Here's how the part is built. I have some questions about the finished solid (model axes, mm). A direction names the side the tool comes from. Give positions to 0.01 mm unless a question says otherwise; leave off trailing zeros. Write each loop counter-clockwise with the first axis right and the second up, starting at its lowest first coordinate (ties: lowest second). Pieces come first, ordered by that corner, then holes. Notation, with made-up numbers: (41, 24.25) - (83, 24.25) arc R24 ccw to (83, 39.25) - close; hole circle Ø11 at (56.25, 40.5). An arc over 180 degrees is marked (long way). Use a Markdown table: item, result.
```python
from build123d import *

# Parameters (mm, degrees)
SKETCH1_R               = 14.95
BOSS_EXTRUDE1_DEPTH     = 14
SKETCH3_R               = 14.95
BOSS_EXTRUDE2_DEPTH     = 14
CHAMFER1_SIZE           = 1
SKETCH11_R              = 11.5
BOSS_EXTRUDE3_DEPTH     = 9
CUT_EXTRUDE1_DEPTH      = 37.465120321
CUT_EXTRUDE1_DEPTH_BACK = 37.465120321
SKETCH9_R               = 7.2
CUT_EXTRUDE2_DEPTH      = 37.465120321
CUT_EXTRUDE2_DEPTH_BACK = 37.465120321
SKETCH10_W              = 2.718236021
SKETCH10_H              = 5.3


with BuildPart() as part:
    # Sketch1 → Boss-Extrude1 (new body)
    with BuildSketch(Plane(origin=(0, 0, 0), x_dir=(1, 0, 0), z_dir=(0, 1, 0))):
        with Locations(Location((0, 0, 0), (0, 0, 270))):
            Circle(SKETCH1_R)
    extrude(amount=BOSS_EXTRUDE1_DEPTH)

    # Sketch3 → Boss-Extrude2 (add)
    with BuildSketch(Plane.XZ):
        with Locations(Location((3, 0, 0), (0, 0, 95.758429808))):
            Circle(SKETCH3_R)
    extrude(amount=BOSS_EXTRUDE2_DEPTH)

    # Chamfer1
    chamfer1_edges = [part.edges().sort_by_distance(p)[0] for p in [
        (0, 14, -14.95),
        (4.5, -14, -14.874558817),
    ]]
    chamfer(chamfer1_edges, length=CHAMFER1_SIZE)

    # Sketch11 → Boss-Extrude3 (add)
    with BuildSketch(Plane(origin=(0, 14, 0), x_dir=(1, 0, 0), z_dir=(0, 1, 0))):
        with Locations(Location((1.5, 0, 0), (0, 0, 270))):
            Circle(SKETCH11_R)
    extrude(amount=BOSS_EXTRUDE3_DEPTH)

    # Sketch9 → Cut-Extrude1 (cut, two sides: drawn at the far end of the back side and taken through both)
    with BuildSketch(Plane(origin=(0, 14, 0), x_dir=(1, 0, 0), z_dir=(0, 1, 0)).offset(-CUT_EXTRUDE1_DEPTH_BACK)):
        with Locations(Location((1.5, 0, 0), (0, 0, 270))):
            Circle(SKETCH9_R)
    extrude(amount=CUT_EXTRUDE1_DEPTH + CUT_EXTRUDE1_DEPTH_BACK, mode=Mode.SUBTRACT)

    # Sketch10 → Cut-Extrude2 (cut, two sides: drawn at the far end of the back side and taken through both)
    with BuildSketch(Plane(origin=(0, 14, 0), x_dir=(1, 0, 0), z_dir=(0, 1, 0)).offset(-CUT_EXTRUDE2_DEPTH_BACK)):
        with Locations((9.14088199, 0)):
            Rectangle(SKETCH10_W, SKETCH10_H)
    extrude(amount=CUT_EXTRUDE2_DEPTH + CUT_EXTRUDE2_DEPTH_BACK, mode=Mode.SUBTRACT)


solid = part.part
```
Item 1: If we section it at A-A, the plane z = 0: Write out the boundary of the cut face in (x, y), plus the area to 3 significant figures.
Values:
| item | result |
|---|---|
| outline | (-14.95, 0) - (-11.95, 0) - (-11.95, -13) - (-10.95, -14) - (-5.7, -14) - (-5.7, 23) - (-10, 23) - (-10, 14) - (-13.95, 14) - (-14.95, 13) - close; (10.5, -14) - (16.95, -14) - (17.95, -13) - (17.95, 0) - (14.95, 0) - (14.95, 13) - (13.95, 14) - (13, 14) - (13, 23) - (10.5, 23) - close |
| area | 443 mm2 |
Item 2: If we section it at B-B, the plane y = 17.5: Write out the boundary of the cut face in (x, z), plus the area to 3 significant figures.
Values:
| item | result |
|---|---|
| outline | circle Ø23 at (1.5, 0); hole (8.19, -2.65) - (10.5, -2.65) - (10.5, 2.65) - (8.19, 2.65) arc R7.2 ccw (long way) to start |
| area | 242 mm2 |
Item 3: I need wall thicknesses on line 1 along X through (y, z) = (9.5, 0); line 2 along Z through (x, y) = (1, 12.5); line 3 along Z through (x, y) = (10, 19). Which ranges of each line are inside material? Lowest first, please. Write a range as [from, to].
Values:
| item | result |
|---|---|
| line 1 | x = [-14.95, -5.7], [10.5, 14.95] |
| line 2 | z = [-14.92, -7.18], [7.18, 14.92] |
| line 3 | z = [-7.75, -2.65], [2.65, 7.75] |
Item 4: If we section it at C-C, the plane y = 4.5: Write out the boundary of the cut face in (x, z).
Values:
| item | result |
|---|---|
| outline | circle Ø29.9 at (0, 0); hole (8.19, -2.65) - (10.5, -2.65) - (10.5, 2.65) - (8.19, 2.65) arc R7.2 ccw (long way) to start |
Item 5: Will these pins go through, and if not, where does the flat tip stop? pin 1 Ø12 at (x, y) = (-6.5, 0.5) entering from +Z; pin 2 Ø10 at (y, z) = (-8, -5.5) entering from -X; pin 3 Ø1 at (y, z) = (10, 2) entering from +X.
Values:
| item | result |
|---|---|
| pin 1 | stops at z = 14.94 |
| pin 2 | stops at x = -11.94 |
| pin 3 | stops at x = 14.87 |
Item 6: For faces 4 (the flat face through (-6, 23, 0)), 5 (the cylindrical face through (11.2, 18.44, 6.18)), 6 (the flat face through (15.1, 0, -1.1)), 7 (the flat face through (-12.2, 0, -0.1)), 8 (the flat face through (10.5, 4, 0)), which set-ups out of +Z, -Z, +X, -X, +Y, -Y let a thin tool reach every point of the face, with its end or its side?
Values:
| item | result |
|---|---|
| face 4 | +Z, -Z, +X, -X, +Y |
| face 5 | +Y |
| face 6 | +X, +Y |
| face 7 | -X, -Y |
| face 8 | +Y, -Y |
Item 7: Thinking about a two-plate mould opening in Z: for faces 1 (the cylindrical face through (13.24, -6.41, -10.89)), 2 (the flat face through (9, -14, 3)), 3 (the cylindrical face through (-5.695, 4.241, -0.279)), which applies, +Z half, -Z half, draft (parallel to the pull), parting line (faces both ways), or undercut?
Values:
| item | result |
|---|---|
| face 1 | parting line |
| face 2 | draft |
| face 3 | undercut |
